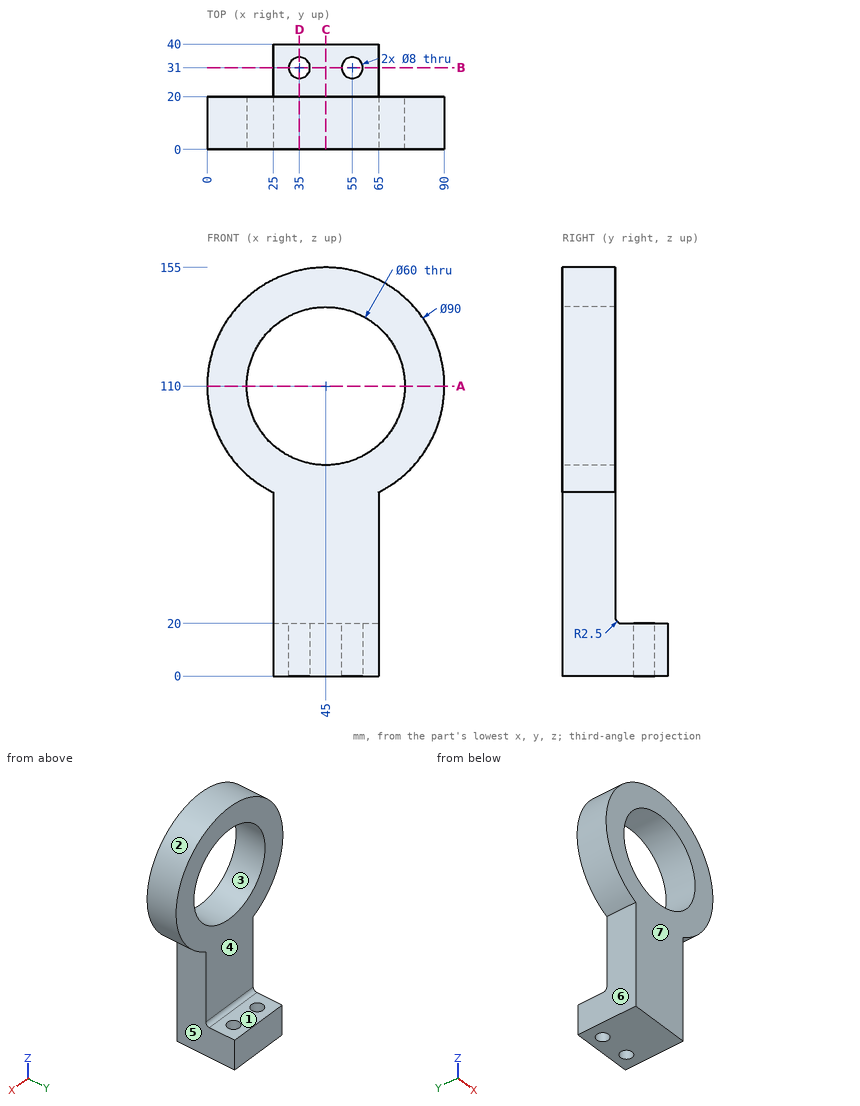
Print and shaded views of the part. All mm, measured from the part's lowest x, y and z. A direction names the side the tool comes from. Round coordinates to 2 decimals unless told otherwise and drop trailing zeros. Write each loop counter-clockwise with the first axis right and the second up, starting at its lowest first coordinate (ties: lowest second). Pieces come first, ordered by that corner, then holes. Notation, with made-up numbers: (77.25, -18) -> (93.25, -18) arc R22 cw to (93.25, -1) -> close; hole circle Ø7 at (-18.5, -12). An arc over 180 degrees is marked (long way). Answer in a Markdown table with one row per item. Add a question column.
Item 1: Mould opens along Z. For the marked faces 1, 2, 3 and 4 say: pulls with the +Z half, pulls with the -Z half, needs draft (parallel to the pull), parting line crosses it, or undercut.
Item 2: Saw through at C-C, the plane x = 45. Write the cut outline in (y, z), then the cut area to 3 significant figures.
Item 3: Saw through at D-D, the plane x = 35. Write the cut outline in (y, z), then the cut area to 3 significant figures.
Item 4: Drill centre lines: line 1 (Z direction, x = 45, y = 4.5); line 2 (X direction, y = 33, z = 15); line 3 (Y direction, x = 55, z = 15). Where is each one in solid material? Low to high. Write a range as from..to.
Item 5: Saw through at A-A, the plane z = 110. Write the cut outline in (x, y), then the cut area to 3 significant figures.
Item 6: Drop flat-ended pins along their axis: pin 1 Ø1 at (x, y) = (10, 15.5) entering from -Z; pin 2 Ø9 at (x, y) = (35, 31) entering from +Z; pin 3 Ø2 at (x, z) = (26, 57.5) entering from +Y; pin 4 Ø12 at (x, z) = (27.5, 90.5) entering from -Y. Give the stop position or say it passes through.
Item 7: Saw through at B-B, the plane y = 31. Write the cut outline in (x, z).
Item 8: Which spindle directions (+Z, -Z, +X, -X, +Y, -Y) get a long thin tool onto all of the face, cutting with end or side? Do the marked faces 5, 6 and 7. Say none if no direction does.
Findings below:
| question | item | result |
|---|---|---|
| 1 | face 1 | pulls with the +Z half |
| 1 | face 2 | parting line crosses it |
| 1 | face 3 | undercut |
| 1 | face 4 | needs draft |
| 2 | outline | (0, 0) -> (40, 0) -> (40, 20) -> (22.5, 20) arc R2.5 cw to (20, 22.5) -> (20, 80) -> (0, 80) -> close; (0, 140) -> (20, 140) -> (20, 155) -> (0, 155) -> close |
| 2 | area | 2,300 mm^2 |
| 3 | outline | (0, 0) -> (27, 0) -> (27, 20) -> (22.5, 20) arc R2.5 cw to (20, 22.5) -> (20, 81.72) -> (0, 81.72) -> close; (0, 138.28) -> (20, 138.28) -> (20, 153.87) -> (0, 153.87) -> close; (35, 0) -> (40, 0) -> (40, 20) -> (35, 20) -> close |
| 3 | area | 2,190 mm^2 |
| 4 | line 1 | z = 0..80, 140..155 |
| 4 | line 2 | x = 25..31.54, 38.46..51.54, 58.46..65 |
| 4 | line 3 | y = 0..27, 35..40 |
| 5 | outline | (0, 0) -> (15, 0) -> (15, 20) -> (0, 20) -> close; (75, 0) -> (90, 0) -> (90, 20) -> (75, 20) -> close |
| 5 | area | 600 mm^2 |
| 6 | pin 1 | stops at z = 81.11 |
| 6 | pin 2 | stops at z = 20 |
| 6 | pin 3 | stops at y = 20 |
| 6 | pin 4 | stops at y = 0 |
| 7 | outline | (25, 0) -> (31, 0) -> (31, 20) -> (25, 20) -> close; (39, 0) -> (51, 0) -> (51, 20) -> (39, 20) -> close; (59, 0) -> (65, 0) -> (65, 20) -> (59, 20) -> close |
| 8 | face 5 | -Z, +X, +Y, -Y |
| 8 | face 6 | -Z, -X, +Y, -Y |
| 8 | face 7 | +Z, -Z, +X, -X, -Y |
